Check sheet for the modelled part. Datum: model origin and axes. Units: mm. A direction names the side the tool comes from. Round coordinates to 2 decimals unless told otherwise and drop trailing zeros. Order: outer loops, then holes, each group sorted by start corner. A loop starts at its lowest first (then second) coordinate and runs counter-clockwise, first axis right, second up. Notation, with made-up numbers: (48, 23) -> (77, 23) arc R17 ccw to (77, 34) -> close; hole circle Ø2 at (51.5, 4.5). An arc over 180 degrees is marked (long way). Answer in a Markdown table with one row per item.
from build123d import *

# Parameters (mm, degrees)
F0_W     = 38.1
F0_H     = 10.16
F2_R     = 12.7
F3_DEPTH = 88.9
F4_DEPTH = 88.9


# Not quite as in the source:
# - a feature names something its author has since deleted; it is built from what else it names


with BuildPart() as f1:
    # F0 (on Front) → F1 (revolve)
    with BuildSketch(Plane.XZ):
        with BuildLine():
            add(Edge.make_bspline(
                [(-147.2955053902, 10.16), (-143.5447688246, 2.570837969), (-131.58254077, 0), (-116.84, 0)],
                knots=[0, 0, 0, 0, 32.1055043345, 32.1055043345, 32.1055043345, 32.1055043345], degree=3))
            Line((-116.84, 0), (-116.84, 10.16))
            Line((-116.84, 10.16), (-147.2955053902, 10.16))
        make_face()
        with Locations((-97.79, 5.08)):
            Rectangle(F0_W, F0_H)
    revolve(axis=Axis((0, 0, 13.0290351808), (0, 0, -1)))

    # F2 (on face) → F3 (join)
    with BuildSketch(Plane.XY.offset(10.16)):
        with Locations((-54.3942935765, 123.0764985085)):
            Circle(F2_R)
        with Locations((54.3942935765, 123.0764985085)):
            Circle(F2_R)
        with Locations((121.978003574, 56.8147908631)):
            Circle(F2_R)
        with Locations((125.2771361136, -49.1679397622)):
            Circle(F2_R)
        with Locations((54.3942935765, -123.0764985085)):
            Circle(F2_R)
        with Locations((-54.3942935765, -123.0764985085)):
            Circle(F2_R)
        with Locations((-121.9781520783, -56.8146452636)):
            Circle(F2_R)
    extrude(amount=F3_DEPTH)

    # F2 (on face) → F4 (join)
    with BuildSketch(Plane.XY.offset(10.16)):
        with Locations((-125.2057118813, 49.2424128206)):
            Circle(F2_R)
    extrude(amount=F4_DEPTH)


solid = f1.part
Item 1: Cross-section at A-A (z = 46). Record the boundary of the cut face in (x, y).
Result sheet:
| item | result |
|---|---|
| outline | circle Ø25.4 at (-125.21, 49.24); circle Ø25.4 at (-121.98, -56.81); circle Ø25.4 at (-54.39, -123.08); circle Ø25.4 at (-54.39, 123.08); circle Ø25.4 at (54.39, -123.08); circle Ø25.4 at (54.39, 123.08); circle Ø25.4 at (121.98, 56.81); circle Ø25.4 at (125.28, -49.17) |
Item 2: Mould release check, pull along Y, two halves, no side actions. Record for faces 1 (the flat face through (125, -49, 99.06)), 2 (the cylindrical face through (-127.959, 36.844, 53.988)), 3 (the cylindrical face through (-57.147, -135.474, 53.988)): pulls with the +Y half, pulls with the -Y half, needs draft (parallel to the pull), parting line crosses it, or undercut.
Result sheet:
| item | result |
|---|---|
| face 1 | needs draft |
| face 2 | undercut |
| face 3 | undercut |
Item 3: Scan lines: line 1 (X direction, y = -126, z = 67.5); line 2 (Y direction, x = 16, z = 9.5); line 3 (X direction, y = -114, z = 92.5). Record each from-to range of solid material in increasing order. Write a range as [from, to].
Result sheet:
| item | result |
|---|---|
| line 1 | x = [-66.75, -42.04], [42.04, 66.75] |
| line 2 | y = [-146.07, -77.1], [77.1, 146.07] |
| line 3 | x = [-63.28, -45.51], [45.51, 63.28] |
Item 4: Depth check by flat-ended pin: P1, Ø10, axis at y = 56.5, z = 31, coming from the -X side; P2, Ø12, axis at x = -75, z = 38.5, coming from the -Y side; P3, Ø1.5, axis at y = -116, z = 62.5, coming from the -X side. Enter the tip coordinate at first touch or a pass-through.
Result sheet:
| item | result |
|---|---|
| P1 | stops at x = -137.7 |
| P2 | passes through |
| P3 | stops at x = -65.41 |
Item 5: Set-up check for faces 4 (the flat face through (-55, -123, 99.06)), 5 (the flat face through (63, -63, 10.16)): record each of +Z, -Z, +X, -X, +Y, -Y from which the full face is reachable in a straight line by a thin tool's end or side.
Result sheet:
| item | result |
|---|---|
| face 4 | +Z, +X, -X, +Y, -Y |
| face 5 | +Z |
